```python
from build123d import *

# Parameters (mm, degrees)
SKETCH_2_R        = 7.94
EXTRUDE_1_DEPTH   = 7.875
EXTRUDE_1_2_DEPTH = 7.875
EXTRUDE_2_DEPTH   = 3.43
SKETCH_6_R        = 3.97
EXTRUDE_4_DEPTH   = 3.34


with BuildPart() as part:
    # Sketch 2 → Extrude 1 (new, symmetric)
    with BuildSketch(Plane.XY):
        with Locations((12.7, 0)):
            Circle(SKETCH_2_R)
    extrude(amount=EXTRUDE_1_DEPTH, both=True)



with BuildPart() as body_2:
    # Sketch 2 → Extrude 1 2 (new, symmetric)
    with BuildSketch(Plane.XY):
        with Locations((-12.7, 0)):
            Circle(SKETCH_2_R)
    extrude(amount=EXTRUDE_1_2_DEPTH, both=True)


with BuildPart() as part_1:
    add(part.part)

    add(body_2.part)  # Extrude 2 merges body 2
    # Sketch 3 → Extrude 2 (add)
    with BuildSketch(Plane.XY.offset(7.875)):
        with BuildLine():
            ThreePointArc((-10.428153415, 11.849174574), (-24.765, 0), (-10.428153415, -11.849174574))
            ThreePointArc((-10.428153415, -11.849174574), (0, -10.8585), (10.428153415, -11.849174574))
            ThreePointArc((10.428153415, -11.849174574), (24.765, 0), (10.428153415, 11.849174574))
            ThreePointArc((10.428153415, 11.849174574), (0, 10.8585), (-10.428153415, 11.849174574))
        make_face()
    extrude(amount=EXTRUDE_2_DEPTH)


with BuildPart() as body_2_2:
    # Sketch 6 → Extrude 4 (new body)
    with BuildSketch(Plane.XY.offset(11.305)):
        with BuildLine():
            ThreePointArc((32.154770058, -17.228648829), (48.987968132, -9.317166623), (38.048309834, 5.725173103))
            ThreePointArc((38.048309834, 5.725173103), (27.701405286, 7.358998688), (17.847242234, 10.911925695))
            ThreePointArc((17.847242234, 10.911925695), (1.014044161, 3.000443489), (11.953702459, -12.041896237))
            ThreePointArc((11.953702459, -12.041896237), (22.300607007, -13.675721822), (32.154770058, -17.228648829))
        make_face()
        with Locations((12.7, 0)):
            Circle(SKETCH_6_R, mode=Mode.SUBTRACT)
        with Locations((37.302012293, -6.316723134)):
            Circle(SKETCH_6_R, mode=Mode.SUBTRACT)
    extrude(amount=EXTRUDE_4_DEPTH)


solid = body_2_2.part
```
The listing builds one solid part. Answer for the finished solid, in the listing's coordinates (mm). Coordinates: 2 decimals unless noted, no trailing zeros. Loops run counter-clockwise (first coordinate to the right, second up) from the corner with the lowest first, then second, coordinate; pieces in that order, holes last. Notation, with made-up numbers: (-29, -12.75) - (-23, -12.75) arc R28 ccw to (-23, 22.25) - close; hole circle Ø6 at (-8.5, -5). An arc over 180 degrees is marked (long way). Use a Markdown table: item, result. Add a question column.
1) The mould has two halves that part along X. Classify faces 1 (the cylindrical face through (8.734, 0.175, 12.952)), 2 (the cylindrical face through (22.16, -13.64, 12.95)), 3 (the cylindrical face through (1.092, 3.287, 12.952)): released by +X, released by -X, zero draft, split by the parting line, or undercut.
2) Given pin 1 (1 mm diameter, centred on y = 1, z = 12, fed in from -X); pin 2 (10 mm diameter, centred on x = 9.5, y = -1, fed in from -Z) (3 decimals); pin 3 (1.5 mm diameter, centred on x = 20, z = 13, fed in from +Y); pin 4 (1.5 mm diameter, centred on y = -13, z = 12, fed in from +X), each flat-ended and moving along its own axis, determine where each tip first touches the part or whether it passes through.
3) Find the intervals of material crossed by line 1 (X direction, y = -3, z = 11.9); line 2 (X direction, y = -9.5, z = 11.65); line 3 (X direction, y = 1.5, z = 13.85), in increasing order.
4) The part is cut by section C-C, the plane z = 13.4. Give the vertices of the cut face in (x, y) (3 decimals).
5) The part is cut by section D-D, the plane y = -13.5. Give the vertices of the cut face in (x, z) (3 decimals), and give its area (3 significant figures).
6) The part is cut by section A-A, the plane x = 12.7. Give the vertices of the cut face in (y, z) (3 decimals), and give its area (3 significant figures).
7) The part is cut by section B-B, the plane y = -8.5. Give the vertices of the cut face in (x, z) (3 decimals).
Here are the results:
| question | item | result |
|---|---|---|
| 1 | face 1 | undercut |
| 1 | face 2 | released by -X |
| 1 | face 3 | split by the parting line |
| 2 | pin 1 | stops at x = 0.65 |
| 2 | pin 2 | stops at z = 11.305 |
| 2 | pin 3 | stops at y = 10.27 |
| 2 | pin 4 | stops at x = 47.81 |
| 3 | line 1 | x = 1.01 to 10.1, 15.3 to 35.12, 39.48 to 48.9 |
| 3 | line 2 | x = 5.26 to 34.93, 39.67 to 48.94 |
| 3 | line 3 | x = 0.73 to 9.02, 16.38 to 46.49 |
| 4 | outline | (11.954, -12.042) arc R55.38 cw to (32.155, -17.229) arc R12.065 ccw (long way) to (38.048, 5.725) arc R55.38 cw to (17.847, 10.912) arc R12.065 ccw (long way) to start; hole circle Ø7.94 at (12.7, 0); hole circle Ø7.94 at (37.302, -6.317) |
| 5 | outline | (21.597, 11.305) - (46.996, 11.305) - (46.996, 14.645) - (21.597, 14.645) - close |
| 5 | area | 84.8 mm^2 |
| 6 | outline | (-12.093, 11.305) - (-3.97, 11.305) - (-3.97, 14.645) - (-12.093, 14.645) - close; (3.97, 11.305) - (12.065, 11.305) - (12.065, 14.645) - (3.97, 14.645) - close |
| 6 | area | 54.2 mm^2 |
| 7 | outline | (4.138, 11.305) - (33.986, 11.305) - (33.986, 14.645) - (4.138, 14.645) - close; (40.618, 11.305) - (49.168, 11.305) - (49.168, 14.645) - (40.618, 14.645) - close |
